from build123d import *

# Parameters (mm, degrees)
SKETCH1_W            = 85
SKETCH1_H            = 41
BOSS_EXTRUDE1_DEPTH  = 5
SKETCH3_W            = 45
SKETCH3_H            = 10
BOSS_EXTRUDE3_DEPTH  = 30
SKETCH4_W            = 6
SKETCH4_H            = 6
SKETCH4_R            = 1.5
BOSS_EXTRUDE4_DEPTH  = 5
LPATTERN1_COUNT      = 2
LPATTERN1_PITCH      = 35
LPATTERN1_COUNT_DIR2 = 2
LPATTERN1_PITCH_DIR2 = 91
FILLET1_R            = 20
SKETCH5_R            = 2.5
CUT_EXTRUDE1_DEPTH   = 41
FILLET2_R            = 1
FILLET3_R            = 10


with BuildPart() as part:
    # Sketch1 → Boss-Extrude1 (new body)
    with BuildSketch(Plane.XY):
        with Locations((42.5, 20.5)):
            Rectangle(SKETCH1_W, SKETCH1_H)
    extrude(amount=BOSS_EXTRUDE1_DEPTH)

    # Sketch3 → Boss-Extrude3 (add)
    with BuildSketch(Plane.XY.offset(5)):
        with Locations((42.5, 36)):
            Rectangle(SKETCH3_W, SKETCH3_H)
        with Locations((42.5, 5)):
            Rectangle(SKETCH3_W, SKETCH3_H)
    extrude(amount=BOSS_EXTRUDE3_DEPTH)

    # Sketch4 → Boss-Extrude4 (add)
    with BuildSketch(Plane.XY.offset(5)):
        with Locations((-3, 38)):
            Rectangle(SKETCH4_W, SKETCH4_H)
        with Locations((-3, 38)):
            Circle(SKETCH4_R, mode=Mode.SUBTRACT)
    boss_extrude4 = extrude(amount=-BOSS_EXTRUDE4_DEPTH)

    # LPattern1: Boss-Extrude4 2 × 2
    with Locations(*[(j * LPATTERN1_PITCH_DIR2, -i * LPATTERN1_PITCH, 0) for i in range(LPATTERN1_COUNT) for j in range(LPATTERN1_COUNT_DIR2) if (i, j) != (0, 0)]):
        add(boss_extrude4)

    # Fillet1
    fillet1_edges = [part.edges().sort_by_distance(p)[0] for p in [
        (20, 36, 5),
        (65, 36, 5),
        (20, 5, 5),
        (65, 5, 5),
    ]]
    fillet(fillet1_edges, radius=FILLET1_R - 0.0001)  # a hair under: the kernel refuses the full size

    # Sketch5 → Cut-Extrude1 (cut)
    with BuildSketch(Plane(origin=(0, 41, 0), x_dir=(1, 0, 0), z_dir=(0, 1, 0))):
        with Locations(Location((30, -25, 0), (0, 0, 270))):
            Circle(SKETCH5_R)
        with Locations(Location((55, -25, 0), (0, 0, 270))):
            Circle(SKETCH5_R)
    extrude(amount=-CUT_EXTRUDE1_DEPTH, mode=Mode.SUBTRACT)

    # Fillet2
    fillet2_edges = [part.edges().sort_by_distance(p)[0] for p in [
        (0, 35, 2.5),
        (85, 35, 2.5),
        (0, 6, 2.5),
        (85, 6, 2.5),
    ]]
    fillet(fillet2_edges, radius=FILLET2_R)

    # Fillet3
    fillet3_edges = [part.edges().sort_by_distance(p)[0] for p in [
        (65, 5, 35),
        (20, 5, 35),
        (65, 36, 35),
        (20, 36, 35),
    ]]
    fillet(fillet3_edges, radius=FILLET3_R)


solid = part.part
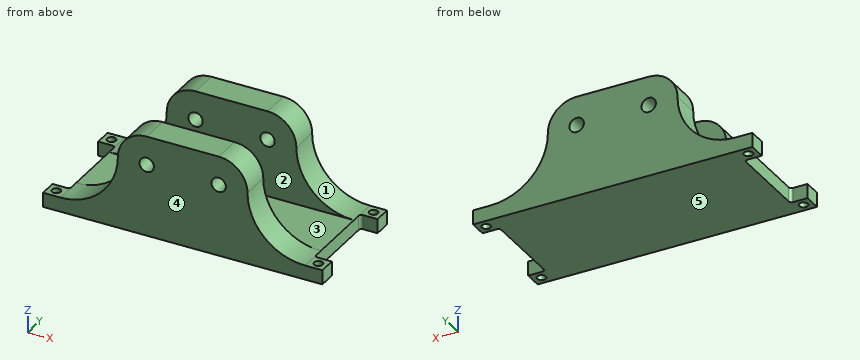
Can you work these out from the model? Positions are in its coordinate system, mm. Face numbers are marked on the shaded views. A direction names the side the tool comes from. Coordinates: 2 decimals unless noted, no trailing zeros. Write each loop counter-clockwise with the first axis right and the second up, starting at its lowest first coordinate (ties: lowest second). Pieces come first, ordered by that corner, then holes. Notation, with made-up numbers: (-19, 82.5) -> (31, 82.5) arc R19 ccw to (31, 97.5) -> close; hole circle Ø11 at (31.25, 64.25). An arc over 180 degrees is marked (long way). Write item = value, one per line.
(1) On a 3-axis mill with a long thin cutter (end or side, diameter ignored), from which of +Z, -Z, +X, -X, +Y, -Y can I reach the whole of each face in a straight line? I mean the marked faces 1 and 2. Say none if no direction works.
Verdict:
face_1 = +Z, +X, +Y, -Y
face_2 = +Z, +X, -X
(2) Imagine slicing it at B-B (z = 4). Please give me the cut outline in (x, y), and give its area (3 significant figures).
Verdict:
outline = (-6, 0) -> (91, 0) -> (91, 6) -> (86, 6) arc R1 cw to (85, 7) -> (85, 34) arc R1 cw to (86, 35) -> (91, 35) -> (91, 41) -> (-6, 41) -> (-6, 35) -> (-1, 35) arc R1 cw to (0, 34) -> (0, 7) arc R1 cw to (-1, 6) -> (-6, 6) -> close; hole circle Ø3 at (-3, 3); hole circle Ø3 at (-3, 38); hole circle Ø3 at (88, 3); hole circle Ø3 at (88, 38)
area = 3,600 mm^2
(3) Imagine slicing it at D-D (x = 40.5). Please give me the cut outline in (y, z), and give its area (3 significant figures).
Verdict:
outline = (0, 0) -> (41, 0) -> (41, 35) -> (31, 35) -> (31, 5) -> (10, 5) -> (10, 35) -> (0, 35) -> close
area = 805 mm^2
(4) Imagine slicing it at A-A (y = 38). State how many separate pieces and enclosed holes the cut face has, and give its area (3 significant figures).
Verdict:
separate_pieces = 3
enclosed_holes = 2
area = 1,890 mm^2
(5) For pin 1 (5 mm diameter, centred on y = 6, z = 15, fed in from -X); pin 2 (3 mm diameter, centred on x = 30, z = 25, fed in from +Y); pin 3 (10 mm diameter, centred on y = 33.5, z = 30.5, fed in from +X); pin 4 (2 mm diameter, centred on x = 13, y = 7, fed in from +Z), each with a flat end and sliding along its axis, tell me the tip position at first contact or that it passes through.
Verdict:
pin_1 = 15.61
pin_2 = through
pin_3 = 64.99
pin_4 = 10.72
(6) If I drill on probe 1 along X at (y, z) = (3.5, 25); probe 2 along Y at (x, z) = (-3, 1.3); probe 3 along Y at (x, z) = (28.5, 17), over which ranges is the centre line in solid material (lowest first)?
Verdict:
probe_1 = 20 to 27.5, 32.5 to 52.5, 57.5 to 65
probe_2 = 0 to 1.5, 4.5 to 6, 35 to 36.5, 39.5 to 41
probe_3 = 0 to 10, 31 to 41
(7) Thinking about a two-plate mould opening in Y: for the marked faces 3, 4 and 5, which applies, +Y half, -Y half, draft (parallel to the pull), parting line (faces both ways), or undercut?
Verdict:
face_3 = undercut
face_4 = -Y half
face_5 = draft
